Model file for the job. Use its own axes, mm. A direction names the side the tool comes from. Round coordinates to 2 decimals unless told otherwise and drop trailing zeros. Order: outer loops, then holes, each group sorted by start corner. A loop starts at its lowest first (then second) coordinate and runs counter-clockwise, first axis right, second up. Notation, with made-up numbers: (-34, 28) -> (-11, 28) arc R26 ccw to (-11, 59) -> close; hole circle Ø4 at (40.25, 70). An arc over 180 degrees is marked (long way). Put each result on its own line as item: value. Start each with the question number.
Q1. Pull direction X, two halves, no side cores. Call faces 1 (the face through (-3.74, 3.13, 16.86)), 2 (the face through (-0.35, 3.131, 50.794)), 3 (the face through (0, 6.35, 20)): released by +X, released by -X, zero draft, split by the parting line, or undercut.
Q2. Flat gauge pins, fed straight in: P1, Ø3, axis at x = -15.5, y = 4.5, coming from the +Z side; P2, Ø12, axis at x = -5, z = 27, coming from the -Y side. Where does each tip first touch, or does it go through?
Q3. Probe L1, parallel to Z at x = -1, y = 6; L2, parallel to Z at x = 8, y = 1; L3, parallel to Z at x = 16.5, y = 0.75. List the from-to ranges inside material, lowest first.
Q4. Cut at A-A, the plane z = 43.5. List the corners of the cut face in (x, y).
Q5. 3-axis set-ups, long thin cutter, end or side, ignore diameter. For faces 4 (the face through (15, 3, 40.64)), 5 (the face through (-0.04, 3.13, -10.16)), 6 (the face through (0.24, 3.13, -20.32)), 7 (the face through (0, 0, 20)), 8 (the face through (-16, 3, 0)): which of +Z, -Z, +X, -X, +Y, -Y reach the whole face in a straight line?
Q6. Cut at C-C, the plane y = 2.25. List the corners of the cut face in (x, z), and give its area (3 significant figures).
Q7. Cut at D-D, the plane z = -3.5. List the corners of the cut face in (x, y).
Q8. Cut at B-B, the plane x = -6. List the corners of the cut face in (y, z), and give its area (3 significant figures).
Autodesk Fusion 360 part; units mm, degrees
sketch "Sketch1" plane through (0, 0, 0) normal (0, 1, 0) x (1, 0, 0)
  line L0 (-19.0076, 0) -> (-12.0684, 0)
  arc A0 (10.16, 0) -> (-10.8108, 1.0933) centre (-0.3734, -0.3734) ccw
  line L1 (0, -40.64) -> (0, -50.8)
  line L2 (19.0076, -40.64) -> (11.3592, -40.64)
  arc A1 (-10.16, -40.64) -> (10.0971, -41.7689) centre (0, -40.64) ccw
  line L3 (-14.3684, -26.2716) -> (7.1842, -7.1842)
  line L4 (-7.1842, -33.4558) -> (14.3684, -14.3684)
  arc A2 (7.1842, -7.1842) -> (10.16, 0) centre (1.2978, -0.5376) ccw
  arc A3 (20.32, 0) -> (-20.2748, 1.3547) centre (0, 0) ccw
  arc A4 (-20.32, -40.64) -> (20.2748, -41.9947) centre (0, -40.64) ccw
  arc A5 (14.3684, -14.3684) -> (20.32, 0) centre (2.5957, -1.0752) ccw
  arc A6 (-7.1842, -33.4558) -> (-10.16, -40.64) centre (-1.2978, -40.1024) ccw
  arc A7 (-14.3684, -26.2716) -> (-20.32, -40.64) centre (0, -40.64) ccw
  arc A8 (20.2748, -41.9947) -> (19.0076, -40.64) centre (19.0076, -41.91) ccw
  arc A9 (11.3592, -40.64) -> (10.0971, -41.7689) centre (11.3592, -41.91) ccw
  arc A10 (-20.2748, 1.3547) -> (-19.0076, 0) centre (-19.0076, 1.27) ccw
  arc A11 (-12.0684, 0) -> (-10.8108, 1.0933) centre (-12.0684, 1.27) ccw
  dimension "d11" = 10.16
  dimension "d15" = 1.27
extrude "Extrude1" add sketch "Sketch1" along normal blind 6.35
Ans:
1. face 1: released by -X
1. face 2: undercut
1. face 3: zero draft
2. P1: stops at z = 55.37
2. P2: stops at y = 0
3. L1: z = -20.3 to -10.15, 14.43 to 27.98, 50.75 to 60.94
3. L2: z = -18.68 to -6.03, 6.36 to 20.01, 46.9 to 59.32
3. L3: z = -11.86 to 12.12, 40.64 to 52.5
4. outline: (-20.12, 0) -> (-9.75, 0) -> (-9.75, 6.35) -> (-20.12, 6.35) -> close; (9.75, 0) -> (20.12, 0) -> (20.12, 6.35) -> (9.75, 6.35) -> close
5. face 4: +X, +Y, -Y
5. face 5: +Y, -Y
5. face 6: -Z, +Y, -Y
5. face 7: +Z, -Z, +X, -X, -Y
5. face 8: -X, +Y, -Y
6. outline: (-20.32, 40.64) arc R20.32 ccw to (-14.37, 26.27) -> (7.18, 7.18) arc R8.88 cw to (10.16, 0) arc R10.54 cw to (-10.81, -1.09) arc R1.27 ccw to (-12.07, 0) -> (-19.01, 0) arc R1.27 ccw to (-20.27, -1.35) arc R20.32 ccw to (20.32, 0) arc R17.76 ccw to (14.37, 14.37) -> (-7.18, 33.46) arc R8.88 cw to (-10.16, 40.64) arc R10.16 cw to (10.1, 41.77) arc R1.27 ccw to (11.36, 40.64) -> (19.01, 40.64) arc R1.27 ccw to (20.27, 41.99) arc R20.32 ccw to start
6. area: 1,500 mm^2
7. outline: (-20.02, 0) -> (-10.18, 0) -> (-10.18, 6.35) -> (-20.02, 6.35) -> close; (9.43, 0) -> (20.02, 0) -> (20.02, 6.35) -> (9.43, 6.35) -> close
8. outline: (0, -19.41) -> (6.35, -19.41) -> (6.35, -8.54) -> (0, -8.54) -> close; (0, 18.86) -> (6.35, 18.86) -> (6.35, 32.41) -> (0, 32.41) -> close; (0, 48.84) -> (6.35, 48.84) -> (6.35, 60.05) -> (0, 60.05) -> close
8. area: 226 mm^2
